Geometry check sheet. Reference: the model listing, model coordinates, mm. Face numbers are marked on the shaded views. Coordinates: 2 decimals unless noted, no trailing zeros. Write each loop counter-clockwise with the first axis right and the second up, starting at its lowest first coordinate (ties: lowest second). Pieces come first, ordered by that corner, then holes. Notation, with made-up numbers: M 25.25,-4 L 47.25,-4 A27 ccw 47.25,32 Z; hole C -15.5,14 d5. An arc over 180 degrees is marked long. Put each result on its own line as item: value. Start each with the question number.
1) Mould release check, pull along Y, two halves, no side actions. Record for the marked faces 1, 2 and 3: released by +Y, released by -Y, zero draft, split by the parting line, or undercut.
2) Scan lines: line 1 along Y through (x, z) = (0, 20.1); line 2 along Y through (x, z) = (0, 6.75); line 3 along X through (y, z) = (3, 18.75). Record each from-to range of solid material in increasing order.
3) Gauge pin test, flat ends, axial feed: pin 1 (4 mm diameter, centred on x = -3.5, z = 15, fed in from -Y); pin 2 (6 mm diameter, centred on x = -5.5, z = 7, fed in from +Y); pin 3 (5 mm diameter, centred on x = -5, z = 18, fed in from -Y). Record the tip position at first contact, or that the pin passes through.
4) Cross-section at A-A on x = 0. Record the cut outline in (y, z).
5) Cross-section at C-C on z = 20. Record the cut outline in (x, y).
6) Cross-section at D-D on z = 12.75. Record the cut outline in (x, y), plus the area to 3 significant figures.
from build123d import *

# Parameters (mm, degrees)
SKETCH_1_R          = 7
EXTRUDE_1_DEPTH     = 16
SKETCH_2_R          = 8.5
EXTRUDE_2_DEPTH     = 6
SKETCH_3_R          = 7.5
CUT_EXTRUDE_1_DEPTH = 4
SKETCH_4_R          = 6
CUT_EXTRUDE_2_DEPTH = 25


with BuildPart() as part:
    # 草图1 → 凸台-拉伸1 (new body)
    with BuildSketch(Plane.XY):
        Circle(SKETCH_1_R)
    extrude(amount=EXTRUDE_1_DEPTH)

    # 草图2 → 凸台-拉伸2 (add)
    with BuildSketch(Plane.XY.offset(16)):
        Circle(SKETCH_2_R)
    extrude(amount=EXTRUDE_2_DEPTH)

    # 草图3 → 切除-拉伸1 (cut)
    with BuildSketch(Plane.XY.offset(22)):
        Circle(SKETCH_3_R)
    extrude(amount=-CUT_EXTRUDE_1_DEPTH, mode=Mode.SUBTRACT)

    # 草图4 → 切除-拉伸2 (cut)
    with BuildSketch(Plane(origin=(0, 0, 0), x_dir=(-1, 0, 0), z_dir=(0, 0, -1))):
        Circle(SKETCH_4_R)
    extrude(amount=-CUT_EXTRUDE_2_DEPTH, mode=Mode.SUBTRACT)


solid = part.part
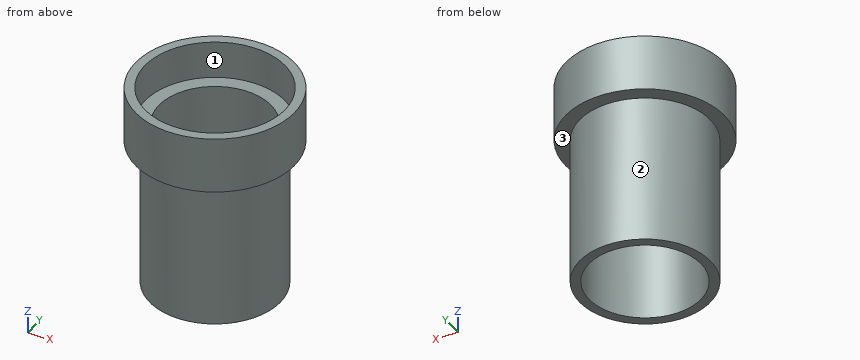
Answer key:
1. face 1: undercut
1. face 2: split by the parting line
1. face 3: zero draft
2. line 1: y = -8.5 to -7.5, 7.5 to 8.5
2. line 2: y = -7 to -6, 6 to 7
2. line 3: x = -7.95 to -6.87, 6.87 to 7.95
3. pin 1: stops at y = -8.31
3. pin 2: stops at y = 6.54
3. pin 3: stops at y = -8.12
4. outline: M -8.5,16 L -7,16 L -7,0 L -6,0 L -6,18 L -7.5,18 L -7.5,22 L -8.5,22 Z; M 6,0 L 7,0 L 7,16 L 8.5,16 L 8.5,22 L 7.5,22 L 7.5,18 L 6,18 Z
5. outline: C 0,0 d17; hole C 0,0 d15
6. outline: C 0,0 d14; hole C 0,0 d12
6. area: 40.8 mm²
